Part model, mm, in its own coordinate system. A direction names the side the tool comes from. Give positions to 0.01 mm unless a question says otherwise; leave off trailing zeros. Order: outer loops, then holes, each group sorted by start corner. A loop starts at its lowest first (then second) coordinate and runs counter-clockwise, first axis right, second up. Notation, with made-up numbers: M 77.5,86 L 125.5,86 A23 ccw 125.5,109 Z; hole C 37.5,36 d3. An arc over 180 degrees is marked long. Return JSON: item names as keys, results as strings.
from build123d import *

# Parameters (mm, degrees)
BOX_W          = 13.37
BOX_H          = 13.37
BOX_DEPTH      = 14
CYLINDER_R     = 11
CYLINDER_DEPTH = 15


with BuildPart() as cube:
    # Box → Box (new body)
    with BuildSketch(Plane(origin=(-6.68, -6.68, 0), x_dir=(1, 0, 0), z_dir=(0, 0, 1))):
        with Locations((6.685, 6.685)):
            Rectangle(BOX_W, BOX_H)
    extrude(amount=BOX_DEPTH)


with BuildPart() as cut:
    # Cylinder → Cylinder (new body)
    with BuildSketch(Plane.XY):
        Circle(CYLINDER_R)
    extrude(amount=CYLINDER_DEPTH)

    # Cut: cut Cube
    add(cube.part, mode=Mode.SUBTRACT)


solid = cut.part
Q1. Band-saw the part on B-B (x = 0). Give the cut face in (y, z).
Established:
{"outline": "M -11,0 L -6.68,0 L -6.68,14 L 6.69,14 L 6.69,0 L 11,0 L 11,15 L -11,15 Z"}
Q2. Band-saw the part on A-A (z = 13). Give the cut face in (x, y), then the cut area to 3 significant figures.
Established:
{"outline": "C 0,0 d22; hole M -6.68,-6.68 L 6.69,-6.68 L 6.69,6.69 L -6.68,6.69 Z", "area": "201 mm²"}
Q3. Band-saw the part on D-D (y = -9.5). Give the cut face in (x, z), then the cut area to 3 significant figures.
Established:
{"outline": "M -5.55,0 L 5.55,0 L 5.55,15 L -5.55,15 Z", "area": "166 mm²"}
Q4. Pin check, flat tips, straight feed: pin 1 (3 mm diameter, centred on x = 5, z = 13, fed in from -Y); pin 2 (1.5 mm diameter, centred on y = 3.5, z = 7.5, fed in from -X); pin 3 (1.5 mm diameter, centred on x = -7, z = 11, fed in from -Y). Stop position of each tip, or through.
Established:
{"pin 1": "stops at y = -10.43", "pin 2": "stops at x = -10.65", "pin 3": "stops at y = -9.05"}
Q5. 3-axis set-ups, long thin cutter, end or side, ignore diameter. For faces 1 (the flat face through (6.69, 0, 7)), 2 (the flat face through (7, 0, 0)): which of +Z, -Z, +X, -X, +Y, -Y reach the whole face in a straight line?
Established:
{"face 1": "-Z", "face 2": "-Z, +X, -X, +Y, -Y"}
Q6. Probe line 1 along Z through (x, y) = (5.5, -3.75); line 2 along X through (y, z) = (1.5, 2.25); line 3 along X through (y, z) = (5.25, 6). List the from-to ranges inside material, lowest first.
Established:
{"line 1": "z = 14 to 15", "line 2": "x = -10.9 to -6.68, 6.69 to 10.9", "line 3": "x = -9.67 to -6.68, 6.69 to 9.67"}
Q7. Two-plate mould, pull along Y, no slides. Class faces 3 (the flat face through (0, 0, 15)), 4 (the cylindrical face through (-2.38, -10.74, 7.4)), 5 (the flat face through (0, -6.68, 7)): +Y half, -Y half, draft (parallel to the pull), parting line (faces both ways), or undercut.
Established:
{"face 3": "draft", "face 4": "parting line", "face 5": "undercut"}
